from build123d import *

# Parameters (mm, degrees)
SKETCH1_R               = 7.8613
SKETCH1_R_2             = 6.858
BOSS_EXTRUDE1_DEPTH     = 2.0066
CUT_EXTRUDE1_DEPTH      = 12.297190754
CUT_EXTRUDE1_DEPTH_BACK = 12.297190754
SKETCH2_W               = 1.0033
SKETCH2_H               = 15.7226
FILLET1_R               = 0.50165
FILLET2_R               = 0.50165


with BuildPart() as part:
    # Sketch1 → Boss-Extrude1 (new body)
    with BuildSketch(Plane.XY):
        Circle(SKETCH1_R)
        Circle(SKETCH1_R_2, mode=Mode.SUBTRACT)
    extrude(amount=-BOSS_EXTRUDE1_DEPTH)

    # Sketch2 → Cut-Extrude1 (cut, two sides: drawn at the far end of the back side and taken through both)
    with BuildSketch(Plane(origin=(0, 0, 0), x_dir=(0, 0, -1), z_dir=(1, 0, 0)).offset(-CUT_EXTRUDE1_DEPTH_BACK)):
        with Locations((1.50495, 0)):
            Rectangle(SKETCH2_W, SKETCH2_H)
    extrude(amount=CUT_EXTRUDE1_DEPTH + CUT_EXTRUDE1_DEPTH_BACK, mode=Mode.SUBTRACT)

    # Fillet1
    fillet1_edges = [part.edges().sort_by_distance(p)[0] for p in [
        (-6.858, 0, -1.0033),
        (-7.8613, 0, 0),
        (-6.858, 0, 0),
    ]]
    fillet(fillet1_edges, radius=FILLET1_R - 0.0001)  # a hair under: the kernel refuses the full size

    # Fillet2
    fillet2_edges = [part.edges().sort_by_distance(p)[0] for p in [
        (-7.8613, 0, -1.0033),
    ]]
    fillet(fillet2_edges, radius=FILLET2_R)


solid = part.part
Source: CAD feature listing. Evaluate the final solid. Frame: model axes, mm. Give positions to 0.01 mm unless a question says otherwise; leave off trailing zeros. Write each loop counter-clockwise with the first axis right and the second up, starting at its lowest first coordinate (ties: lowest second). Pieces come first, ordered by that corner, then holes. Notation, with made-up numbers: M 19.5,70.5 L 35.5,70.5 A27 cw 35.5,99.5 Z; hole C 57,-15.5 d2. An arc over 180 degrees is marked long. Return JSON: item names as keys, results as strings. Group by question number.
1) First-contact query: pin 1 Ø5 at (x, y) = (-2.5, -4) entering from +Z. Flat tip, straight axial feed; report the tip coordinate or a pass-through.
2) Ray query, L1, parallel to Y at x = 0, z = -0.45; L2, parallel to Y at x = 4, z = -0.5; L3, parallel to X at y = 4.5, z = -0.25. Return the intervals inside material, ascending.
3) Cut plane C-C, the plane z = -0.3. Output: boundary loops of the cut face in (x, y).
Data:
{
 "1": {"pin 1": "stops at z = -0.02"},
 "2": {"L1": "y = -7.86 to -6.86, 6.86 to 7.86", "L2": "y = -6.77 to -5.57, 5.57 to 6.77", "L3": "x = -6.36 to -5.26, 5.26 to 6.36"},
 "3": {"outline": "C 0,0 d15.64; hole C 0,0 d13.8"}
}
